For this review, take the finished solid that the model builds, in its own axes (mm). Face numbers are marked on the shaded views. A direction names the side the tool comes from. Coordinates: 2 decimals unless noted, no trailing zeros. Loops run counter-clockwise (first coordinate to the right, second up) from the corner with the lowest first, then second, coordinate; pieces in that order, holes last. Notation, with made-up numbers: (85.25, 38.25) - (140.25, 38.25) arc R12 ccw to (140.25, 51.25) - close; hole circle Ø3 at (41, 46). An arc over 180 degrees is marked (long way). Use one line per item in the form item = value. Start each with the question number.
1. To check wall thickness, follow probe 1 along X at (y, z) = (1.4, 0); probe 2 along X at (y, z) = (-0.4, 0); probe 3 along Y at (x, z) = (-3.5, -2). State the ranges of each line that lie inside material, in increasing order.
2. Add section A-A on y = 1.5. Give the boundary of the cut face in (x, z), and give its area (3 significant figures).
3. For pin 1 Ø0.8 at (y, z) = (-0.5, -1.5) entering from -X, flat-tipped, find the tip position at first contact; note if it passes through.
4. Add section B-B on z = 0.75. Give the boundary of the cut face in (x, y).
5. Add section D-D on x = -3.5. Give the boundary of the cut face in (y, z), and give its area (3 significant figures).
6. Add section C-C on y = -0.4. Give the boundary of the cut face in (x, z), and give its area (3 significant figures).
7. Machinability: for the marked faces 1, 2, 3, 4 and 5, which of the approach directions +Z, -Z, +X, -X, +Y, -Y give a long, thin tool a straight path to every point of the face, cutting with its end or side? Answer none if there is none.
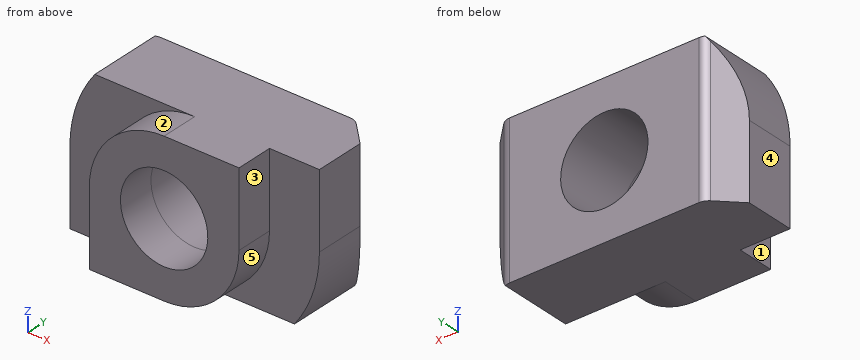
```python
from build123d import *

# Parameters (mm, degrees)
EXTRUDE_1_DEPTH     = 3
SKETCH_2_R          = 1.75
EXTRUDE_2_DEPTH     = 1.5
SKETCH_2_2_R        = 1.75
CUT_EXTRUDE_1_DEPTH = 7.557438524
CUT_EXTRUDE_2_DEPTH = 7.557438524
FILLET_1_R          = 0.5


with BuildPart() as part:
    # Sketch 1 → Extrude 1 (new, symmetric)
    with BuildSketch(Plane.XY):
        Polygon((4, 3), (5, 2), (5, 0), (0, 0), (0, 3), align=None)
    extrude_1 = extrude(amount=EXTRUDE_1_DEPTH, both=True)

    # Mirror 1: Extrude 1 across plane
    add(extrude_1.mirror(Plane(origin=(0, 0, 0), x_dir=(0, 0, 1), z_dir=(1, 0, 0))))

    # Sketch 2 → Extrude 2 (add)
    with BuildSketch(Plane.XZ):
        with BuildLine():
            Line((0, -3), (-3, -3))
            Line((-3, -3), (-3, 0))
            ThreePointArc((-3, 0), (-2.121320344, 2.121320344), (0, 3))
            Line((0, 3), (3, 3))
            Line((3, 3), (3, 0))
            ThreePointArc((3, 0), (2.121320344, -2.121320344), (0, -3))
        make_face()
        with Locations(Location((0, 0, 0), (0, 0, 270))):
            Circle(SKETCH_2_R, mode=Mode.SUBTRACT)
    extrude(amount=EXTRUDE_2_DEPTH)

    # Sketch 2_2 → Cut-Extrude 1 (cut, through all)
    with BuildSketch(Plane.XZ):
        with Locations(Location((0, 0, 0), (0, 0, 270))):
            Circle(SKETCH_2_2_R)
    extrude(amount=-CUT_EXTRUDE_1_DEPTH, mode=Mode.SUBTRACT)

    # Sketch 3 → Cut-Extrude 2 (cut, through all)
    with BuildSketch(Plane.XZ):
        with BuildLine():
            Line((8.00916489, 0), (5, 0))
            ThreePointArc((5, 0), (3.535533906, -3.535533906), (0, -5))
            Line((0, -5), (0, -5.722939185))
            Line((0, -5.722939185), (8.00916489, -5.722939185))
            Line((8.00916489, -5.722939185), (8.00916489, 0))
        make_face()
        with BuildLine():
            Line((-8.00916489, 0), (-5, 0))
            Line((-5, 0), (-5, 3))
            Line((-5, 3), (-4, 3))
            ThreePointArc((-4, 3), (-2.236067977, 4.472135955), (0, 5))
            Line((0, 5), (0, 5.722939185))
            Line((0, 5.722939185), (-8.00916489, 5.722939185))
            Line((-8.00916489, 5.722939185), (-8.00916489, 0))
        make_face()
        with BuildLine():
            Line((-5, 3), (-5, 0))
            ThreePointArc((-5, 0), (-4.74341649, 1.58113883), (-4, 3))
            Line((-4, 3), (-5, 3))
        make_face()
    extrude(amount=-CUT_EXTRUDE_2_DEPTH, mode=Mode.SUBTRACT)

    # Fillet 1
    fillet_1_edges = [part.edges().sort_by_distance(p)[0] for p in [
        (4, 3, 0),
        (-4, 3, 0),
    ]]
    fillet(fillet_1_edges, radius=FILLET_1_R)


solid = part.part
```
Conclusion:
q1.probe_1 = -5 to -1.75, 1.75 to 5
q1.probe_2 = -3 to -1.75, 1.75 to 3
q1.probe_3 = 0 to 3
q2.outline = (-5, -3) - (4, -3) arc R5 ccw to (5, 0) - (5, 3) - (-4, 3) arc R5 ccw to (-5, 0) - close; hole circle Ø3.5 at (0, 0)
q2.area = 48.5 mm^2
q3.pin_1 = -3
q4.outline = (-4.94, 0) - (-2.9, 0) - (-2.9, -1.5) - (-1.58, -1.5) - (-1.58, 3) - (-3.79, 3) arc R0.5 ccw to (-4.15, 2.85) - (-4.94, 2.06) - close; (1.58, -1.5) - (3, -1.5) - (3, 0) - (5, 0) - (5, 2) - (4.15, 2.85) arc R0.5 ccw to (3.79, 3) - (1.58, 3) - close
q5.outline = (0, -3) - (3, -3) - (3, 3) - (0, 3) - close
q5.area = 18.0 mm^2
q6.outline = (-3, -3) - (0, -3) arc R3 ccw to (3, 0) - (3, 3) - (0, 3) arc R3 ccw to (-3, 0) - close; hole circle Ø3.5 at (0, 0)
q6.area = 22.5 mm^2
q7.face_1 = +Z, -Z, -X, -Y
q7.face_2 = +Z, -X, -Y
q7.face_3 = +Z, -Z, +X, -Y
q7.face_4 = +Z, -Z, -X, +Y, -Y
q7.face_5 = -Z, +X, -Y
